Answer from the drawing. Dimensions are ordinates in mm from the lowest x, y and z of the part. A direction names the side the tool comes from. Give positions to 0.01 mm unless a question says otherwise; leave off trailing zeros. Write each loop counter-clockwise with the first axis right and the second up, starting at its lowest first coordinate (ties: lowest second). Pieces come first, ordered by that corner, then holes. Notation, with made-up numbers: M 89.25,87 L 119.25,87 A37 ccw 119.25,123 Z; hole C -33.75,72 d10. An arc over 180 degrees is marked long. Answer as a JSON object with one key per item and string values.
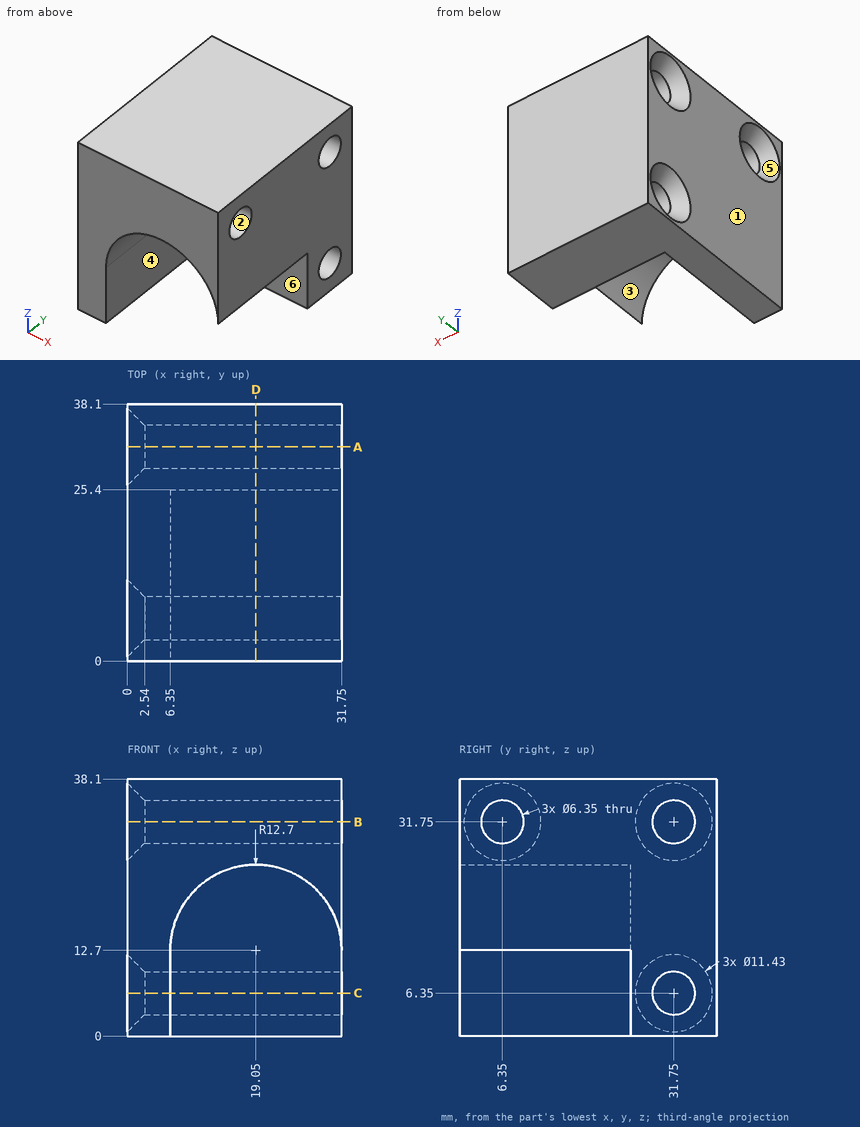
1. A cutting plane is placed at A-A, the plane y = 31.75. Give the vertices of the cut face in (x, z) (3 decimals), plus the area to 3 significant figures.
Verdict:
{"outline": "M 0,0 L 31.75,0 L 31.75,3.175 L 2.54,3.175 L 0,0.635 Z; M 0,12.065 L 2.54,9.525 L 31.75,9.525 L 31.75,28.575 L 2.54,28.575 L 0,26.035 Z; M 0,37.465 L 2.54,34.925 L 31.75,34.925 L 31.75,38.1 L 0,38.1 Z", "area": "794 mm2"}
2. A cutting plane is placed at D-D, the plane x = 19.05. Give the vertices of the cut face in (y, z) (3 decimals), plus the area to 3 significant figures.
Verdict:
{"outline": "M 0,25.4 L 25.4,25.4 L 25.4,0 L 38.1,0 L 38.1,38.1 L 0,38.1 Z; hole C 6.35,31.75 d6.35; hole C 31.75,6.35 d6.35; hole C 31.75,31.75 d6.35", "area": "711 mm2"}
3. The mould has two halves that part along X. Classify the marked faces 1, 2 and 3: released by +X, released by -X, zero draft, split by the parting line, or undercut.
Verdict:
{"face 1": "released by -X", "face 2": "zero draft", "face 3": "undercut"}
4. For the marked faces 4, 5 and 6, determine the directions among +Z, -Z, +X, -X, +Y, -Y from which every point of the face is accessible in a straight line to the end or side of a thin tool.
Verdict:
{"face 4": "-Z, +X, -Y", "face 5": "-X", "face 6": "-Z, -Y"}
5. A cutting plane is placed at C-C, the plane z = 6.35. Give the vertices of the cut face in (x, y) (3 decimals).
Verdict:
{"outline": "M 0,0 L 6.35,0 L 6.35,25.4 L 31.75,25.4 L 31.75,28.575 L 2.54,28.575 L 0,26.035 Z; M 0,37.465 L 2.54,34.925 L 31.75,34.925 L 31.75,38.1 L 0,38.1 Z"}
6. Consider line 1 along Z through (x, y) = (16.5, 31.75) (3 decimals); line 2 along Y through (x, z) = (12, 31). Determine where each line is inside the solid, lowest interval first.
Verdict:
{"line 1": "z = 0 to 3.175, 9.525 to 28.575, 34.925 to 38.1", "line 2": "y = 0 to 3.26, 9.44 to 28.66, 34.84 to 38.1"}
7. Flat-ended cylindrical pins translate along their axes: pin 1 (10 mm diameter, centred on y = 31.75, z = 6.35, fed in from -X) (3 decimals); pin 2 (12.5 mm diameter, centred on x = 16.5, z = 18.5, fed in from -Y); pin 3 (5.5 mm diameter, centred on y = 31.75, z = 31.75, fed in from -X); pin 4 (8.5 mm diameter, centred on y = 6.35, z = 31.75, fed in from -X) (3 decimals). Find the tip coordinate at first contact, or state that the pin passes through.
Verdict:
{"pin 1": "stops at x = 0.715", "pin 2": "stops at y = 25.4", "pin 3": "passes through", "pin 4": "stops at x = 1.465"}
